Work out the finished part from the listing and answer in its coordinate system (mm). A direction names the side the tool comes from. Round coordinates to 2 decimals unless told otherwise and drop trailing zeros. Loops run counter-clockwise (first coordinate to the right, second up) from the corner with the lowest first, then second, coordinate; pieces in that order, holes last.
```python
from build123d import *

# Parameters (mm, degrees)
SKETCH1_W           = 203.2
SKETCH1_H           = 203.2
BOSS_EXTRUDE1_DEPTH = 6.35
CUT_EXTRUDE1_DEPTH  = 7.35
SKETCH9_R           = 3.175
SKETCH9_R_2         = 3.160008279
SKETCH9_R_3         = 3.205750029
SKETCH9_W           = 6.35
SKETCH9_H           = 62.924217451
CUT_EXTRUDE2_DEPTH  = 7.35


with BuildPart() as part:
    # Sketch1 → Boss-Extrude1 (new body)
    with BuildSketch(Plane(origin=(0, 0, 0), x_dir=(1, 0, 0), z_dir=(0, 1, 0))):
        Rectangle(SKETCH1_W, SKETCH1_H)
    extrude(amount=BOSS_EXTRUDE1_DEPTH)

    # Sketch2 → Cut-Extrude1 (cut, through all)
    with BuildSketch(Plane(origin=(0, 6.35, 0), x_dir=(1, 0, 0), z_dir=(0, 1, 0))):
        with BuildLine():
            Line((101.6, 38.1), (101.6, 101.6))
            Line((101.6, 101.6), (38.1, 101.6))
            ThreePointArc((38.1, 101.6), (83.001280605, 83.001280605), (101.6, 38.1))
        make_face()
        with BuildLine():
            Line((-38.1, 101.6), (-101.6, 101.6))
            Line((-101.6, 101.6), (-101.6, 38.1))
            ThreePointArc((-101.6, 38.1), (-83.001280605, 83.001280605), (-38.1, 101.6))
        make_face()
    extrude(amount=-CUT_EXTRUDE1_DEPTH, mode=Mode.SUBTRACT)

    # Sketch9 → Cut-Extrude2 (cut, through all)
    with BuildSketch(Plane.XZ):
        with Locations((-25.490256121, -31.45083867)):
            Circle(SKETCH9_R)
        with Locations((25.309743879, -31.45083867)):
            Circle(SKETCH9_R)
        with Locations((-25.490256121, -76.66283867)):
            Circle(SKETCH9_R)
        with Locations((25.309743879, -76.66283867)):
            Circle(SKETCH9_R)
        with Locations((-47.746294791, 80.015705209)):
            Circle(SKETCH9_R)
        with Locations((-92.71, 80.015705209)):
            Circle(SKETCH9_R)
        with Locations((-47.746294791, 35.052)):
            Circle(SKETCH9_R_2)
        with Locations((-92.71, 35.052)):
            Circle(SKETCH9_R_3)
        with Locations((47.565782549, 80.015705209)):
            Circle(SKETCH9_R)
        with Locations((92.529487758, 80.015705209)):
            Circle(SKETCH9_R)
        with Locations((47.565782549, 35.052)):
            Circle(SKETCH9_R)
        with Locations((92.529487758, 35.052)):
            Circle(SKETCH9_R)
        with Locations((-35.33703867, 42.293852605)):
            Rectangle(SKETCH9_W, SKETCH9_H)
        with Locations((35.156526428, 42.293852605)):
            Rectangle(SKETCH9_W, SKETCH9_H)
    extrude(amount=-CUT_EXTRUDE2_DEPTH, mode=Mode.SUBTRACT)


solid = part.part
```
1. Find section C-C (y = 4.75). Give the number of separate pieces and of enclosed holes in the cut face, then the cut area to 3 significant figures.
Answer key:
separate pieces: 1
enclosed holes: 14
area: 38,400 mm2
2. Which of the six approach directions +Z, -Z, +X, -X, +Y, -Y give full straight-line access (tool end or side, diameter ignored) to faces 4 (the face through (-1, 6.35, -1)), 5 (the face through (35, 3, 73.756))?
Answer key:
face 4: +Z, -Z, +X, -X, +Y
face 5: +Y, -Y
3. Given pin 1 (1 mm diameter, centred on y = 2.5, z = -44.5, fed in from +X), flat-ended and moving along its own axis, determine where the tip first touches the part or whether it passes through.
Answer key:
pin 1: stops at x = 101.33
4. Find section D-D (z = -60). Write down the section's boundary in (x, y).
Answer key:
outline: (-97.7, 0) - (97.7, 0) - (97.7, 6.35) - (-97.7, 6.35) - close
5. Consider probe 1 along X at (y, z) = (6, 18.5); probe 2 along X at (y, z) = (1.5, -33.5); probe 3 along Z at (x, y) = (92.5, 3.75) (3 decimals). Determine where each line is inside the solid, lowest interval first.
Answer key:
probe 1: x = -101.6 to -38.51, -32.16 to 31.98, 38.33 to 101.6
probe 2: x = -101.6 to -27.92, -23.07 to 22.88, 27.73 to 101.6
probe 3: z = -70.855 to 31.877, 38.227 to 76.841, 83.191 to 101.6
6. Determine the mould class of faces 1 (the face through (-1, 3, -101.6)), 2 (the face through (-101.6, 3, 33)), 3 (the face through (95.558, 3.131, 36.006)) for opening direction X: +X half, -X half, draft (parallel to the pull), parting line (faces both ways), or undercut.
Answer key:
face 1: draft
face 2: -X half
face 3: undercut
7. Find section A-A (z = 19). Write down the section's boundary in (x, y).
Answer key:
outline: (-101.6, 0) - (-38.51, 0) - (-38.51, 6.35) - (-101.6, 6.35) - close; (-32.16, 0) - (31.98, 0) - (31.98, 6.35) - (-32.16, 6.35) - close; (38.33, 0) - (101.6, 0) - (101.6, 6.35) - (38.33, 6.35) - close
8. Find section B-B (x = -92.71). Write down the section's boundary in (y, z).
Answer key:
outline: (0, -70.5) - (6.35, -70.5) - (6.35, 31.85) - (0, 31.85) - close; (0, 38.26) - (6.35, 38.26) - (6.35, 76.84) - (0, 76.84) - close; (0, 83.19) - (6.35, 83.19) - (6.35, 101.6) - (0, 101.6) - close
